Verification items for the finished model (mm, model axes). A direction names the side the tool comes from. Coordinates: 2 decimals unless noted, no trailing zeros. Write each loop counter-clockwise with the first axis right and the second up, starting at its lowest first coordinate (ties: lowest second). Pieces come first, ordered by that corner, then holes. Notation, with made-up numbers: (79.5, 3) -> (126.5, 3) arc R16 ccw to (126.5, 11) -> close; hole circle Ø3 at (26, -33.75). An arc over 180 degrees is marked (long way). Write item = value, one per line. Start each with the question number.
(1) Section check D-D (y = 39). Record the cut outline in (x, z), plus the area to 3 significant figures.
(2) Section check A-A (x = -52.5). Record the cut outline in (y, z), plus the area to 3 significant figures.
(3) Mould release check, pull along Z, two halves, no side actions. Record for faces 5 (the face through (-202.03, 52.85, -78.01)), 6 (the face through (-200.99, 22.62, 1.15)), 7 (the face through (-101, 99, -120)), 8 (the face through (-20.1, 50, 0.5)): released by +Z, released by -Z, zero draft, split by the parting line, or undercut.
(4) Gauge pin test, flat ends, axial feed: pin 1 Ø4.5 at (x, z) = (-201.5, -59.5) entering from +Y; pin 2 Ø1.2 at (y, z) = (112, 2.5) entering from -X; pin 3 Ø3 at (x, z) = (-64.5, -89) entering from +Y. Record the tip position at first contact, or that the pin passes through.
(5) Material ranges on probe 1 along Z at (x, y) = (-104, 81); probe 2 along X at (y, z) = (20.5, -107); probe 3 along Y at (x, z) = (-123, -81), recorded low to high. Write a range as [from, to].
(6) Set-up check for faces 1 (the face through (-71.99, 52.85, 1.97)), 2 (the face through (1.97, 147.15, -71.99)), 3 (the face through (-3.01, 25.35, -2.85)), 4 (the face through (-25, 7.9, -120.2)): record each of +Z, -Z, +X, -X, +Y, -Y from which the full face is reachable in a straight line by a thin tool's end or side.
(7) Section check C-C (y = 11). Record the cut outline in (x, z).
(8) Section check B-B (y = 94). Record the cut outline in (x, z).
Autodesk Inventor part; units mm, degrees
ref_plane "YZ Plane" through (0, 0, 0) normal (1, 0, 0) x (0, 1, 0)
ref_plane "XZ Plane" through (0, 0, 0) normal (0, 1, 0) x (-1, 0, 0)
ref_plane "XY Plane" through (0, 0, 0) normal (0, 0, 1) x (1, 0, 0)
sketch "Sketch1" plane through (0, 0, 0) normal (0, 1, 0) x (-1, 0, 0)
  line L0 (0, 0) -> (0, -120)
  line L1 (0, 0) -> (200, 0)
  line L2 (200, 0) -> (200, -120)
  line L3 (200, -120) -> (0, -120)
  dimension "d0" = 120
  dimension "d1" = 200
extrude "Extrusion1" add sketch "Sketch1" along normal blind 200
shell "Shell1" thickness 4 outward yes removed faces 1 at (-66.6667, 200, -40)
sketch "Sketch2" plane through (4, -4, 4) normal (1, 0, 0) x (0, 0, -1)
  line L0 (0, 0) -> (0, 204)
  line L1 (0, 0) -> (0, 204)
  line L2 (4, 4) -> (4, 104)
  line L3 (4, 4) -> (4, 204)
  line L4 (4, 54) -> (124, 54)
  line L5 (124, 4) -> (124, 204)
  line L6 (64, 54) -> (4, 54)
  line L7 (124, 54) -> (64, 54)
  line L8 (94, 54) -> (34, 54)
  line L9 (34, 54) -> (64, 54)
  line L10 (64, 54) -> (94, 54)
  line L11 (79, 54) -> (49, 54)
  line L12 (124, 104) -> (124, 204)
  line L13 (79, 154) -> (49, 154)
  line L14 (79, 54) -> (79, 154)
  line L15 (49, 54) -> (49, 154)
  line L16 (4, 54) -> (4, 204)
  line L17 (4, 204) -> (124, 204)
  line L18 (0, 204) -> (128, 204)
  line L19 (124, 204) -> (124, 54)
extrude "Extrusion2" cut sketch "Sketch2" against normal through all contours L2 L3 L17 L5 L4 L14 L13 L15
sketch "Sketch3" plane through (-204, -4, 4) normal (0, 0, 1) x (1, 0, 0)
  line L0 (204, 54) -> (204, 154)
  line L1 (4, 4) -> (4, 54)
  line L2 (204, 54) -> (4, 54)
  line L3 (4, 54) -> (104, 54)
  line L4 (104, 54) -> (4, 54)
  line L5 (104, 54) -> (54, 54)
  line L6 (208, 54) -> (204, 54)
  line L7 (104, 54) -> (204, 54)
  line L8 (204, 54) -> (154, 54)
  line L9 (154, 54) -> (104, 54)
  line L10 (104, 54) -> (54, 54)
  line L11 (79, 54) -> (129, 54)
  line L12 (129, 154) -> (79, 154)
  line L13 (129, 54) -> (129, 154)
  line L14 (79, 54) -> (79, 154)
  line L15 (4, 54) -> (4, 204)
  line L16 (208, 204) -> (0, 204)
  line L17 (204, 54) -> (204, 204)
  line L18 (4, 54) -> (0, 54)
  line L19 (0, 0) -> (0, 204)
  line L20 (0, 204) -> (0, 54)
  line L21 (0, 204) -> (208, 204)
  line L22 (208, 154) -> (208, 54)
  line L23 (208, 0) -> (208, 204)
  line L24 (208, 54) -> (208, 204)
  line L25 (204, 54) -> (208, 54)
  point P0 (204, 4)
extrude "Extrusion3" cut sketch "Sketch3" against normal blind 10 contours L2 L13 L12 L14 L15 L16 L17 L0 | L0 L17 L16 L23 L22 L6 | L15 L18 L19 L16
sketch "Sketch4" plane through (0, 200, 0) normal (0, 1, 0) x (1, 0, 0)
  point P0 (0, 0)
fillet "Fillet1" radius 10 18 edges at (2, 50, -45) (2, 50, -75) (2, 50, -120) (-202, 50, -120) (-75, 50, 2) (-125, 50, 2) (-202, 50, -45) (-202, 50, -75) (2, 150, -45) (2, 150, -75) (-75, 150, 2) (-125, 150, 2) (-202, 150, -45) (-202, 150, -75) (0, 25, 0) (-200, 25, 0) (-204, 23, 4) (4, 23, 4)
sketch "Sketch5" plane through (4, -4, -124) normal (0, 0, -1) x (-1, 0, 0)
  line L0 (194, 4) -> (4, 4)
  line L1 (204, 4) -> (104, 4)
  line L2 (79, 4) -> (104, 4)
  line L3 (29, 4) -> (4, 4)
  line L4 (79, 4) -> (29, 4)
  line L5 (29, 4) -> (29, 34)
  line L6 (79, 4) -> (79, 34)
  line L7 (79, 34) -> (29, 34)
  line L8 (29, 4) -> (29, 0)
  line L9 (198, 0) -> (10, 0)
  line L10 (29, 0) -> (79, 0)
  line L11 (79, 0) -> (79, 4)
  line L12 (4, 4) -> (29, 4)
  line L13 (79, 4) -> (204, 4)
  line L14 (4, 4) -> (29, 4)
  line L15 (79, 4) -> (104, 4)
  dimension "d10" = 30
extrude "Extrusion4" cut sketch "Sketch5" against normal blind 10
sketch "Sketch6" plane through (0, -4, 0) normal (0, -1, 0) x (1, 0, 0)
  line L0 (-25, -114) -> (-25, -124)
  line L1 (-25, -124) -> (-25, -94)
  line L2 (-75, -124) -> (-75, -94)
  line L3 (-75, -94) -> (-25, -94)
  line L4 (-25, -124) -> (-75, -124)
  line L5 (-25, -124) -> (-75, -124)
  point P0 (0, 0)
  dimension "d13" = 30
extrude "Extrusion5" cut sketch "Sketch6" against normal blind 10
properties part number "bag"
Response:
q1.outline = (-204, -124) -> (4, -124) -> (4, -6) arc R10 ccw to (-6, 4) -> (-194, 4) arc R10 ccw to (-204, -6) -> close; hole (-200, -120) -> (0, -120) -> (0, -10) arc R10 ccw to (-10, 0) -> (-190, 0) arc R10 ccw to (-200, -10) -> close
q1.area = 2,620 mm2
q2.outline = (-4, -94) -> (0, -94) -> (0, 0) -> (50, 0) -> (50, 4) -> (-4, 4) -> close; (30, -124) -> (200, -124) -> (200, -120) -> (30, -120) -> close
q2.area = 1,270 mm2
q3.face_5 = undercut
q3.face_6 = released by +Z
q3.face_7 = undercut
q3.face_8 = zero draft
q4.pin_1 = 150
q4.pin_2 = -125
q4.pin_3 = 0
q5.probe_1 = [-124, -120], [0, 4]
q5.probe_2 = [-204, -200], [0, 4]
q5.probe_3 = [-4, 0]
q6.face_1 = +Z, +X, +Y
q6.face_2 = +X, -X, +Y
q6.face_3 = +Y
q6.face_4 = -Z, -Y
q7.outline = (-204, -124) -> (-75, -124) -> (-75, -120) -> (-200, -120) -> (-200, -10) arc R10 cw to (-190, 0) -> (-10, 0) arc R10 cw to (0, -10) -> (0, -120) -> (-25, -120) -> (-25, -124) -> (4, -124) -> (4, -6) arc R10 ccw to (-6, 4) -> (-194, 4) arc R10 ccw to (-204, -6) -> close
q8.outline = (-204, -124) -> (4, -124) -> (4, -120) -> (-204, -120) -> close; (-204, -75) -> (-200, -75) -> (-200, -45) -> (-204, -45) -> close; (-125, 0) -> (-75, 0) -> (-75, 4) -> (-125, 4) -> close; (0, -75) -> (4, -75) -> (4, -45) -> (0, -45) -> close
